Work out the finished part from the listing and answer in its coordinate system (mm). Face numbers are marked on the shaded views. A direction names the side the tool comes from. Coordinates: 2 decimals unless noted, no trailing zeros. Order: outer loops, then holes, each group sorted by start corner. A loop starts at its lowest first (then second) coordinate and runs counter-clockwise, first axis right, second up. Notation, with made-up numbers: (89, -35.5) -> (121, -35.5) arc R7 ccw to (121, -23.5) -> close; hole circle Ø5 at (42.25, 70.25). An arc over 180 degrees is marked (long way). Write item = value, one per line. Start each with the question number.
Q1. For a pull along Y with two mould halves and no side action, classify the marked faces 1, 2 and 3 as +Y half, -Y half, draft (parallel to the pull), parting line (faces both ways), or undercut.
Q2. The part is cut by section C-C, the plane x = 7.5. Count the separate pieces of the cut face and the enclosed holes in it, plus the area to 3 significant figures.
Q3. The part is cut by section A-A, the plane y = -13.5. Determine the outline of the cut face in (x, z).
Q4. Flat-ended cylindrical pins translate along their axes: pin 1 (6 mm diameter, centred on y = -32.5, z = -13, fed in from +X); pin 2 (3 mm diameter, centred on x = 7, y = -23.5, fed in from -Z). Find the tip coordinate at first contact, or state that the pin passes through.
Q5. The part is cut by section B-B, the plane y = -24. Determine the outline of the cut face in (x, z).
Q6. Which of the six approach directions +Z, -Z, +X, -X, +Y, -Y give full straight-line access (tool end or side, diameter ignored) to the marked faces 4, 5 and 6?
Q7. Straight lines are drawn through the part: L1, parallel to X at y = -25, z = -27.75; L2, parallel to Y at x = 7.5, z = -27.25; L3, parallel to Y at x = 8.5, z = -26.5. For each, find the intervals that lie inside material, in ascending order. Write a range as from..to.
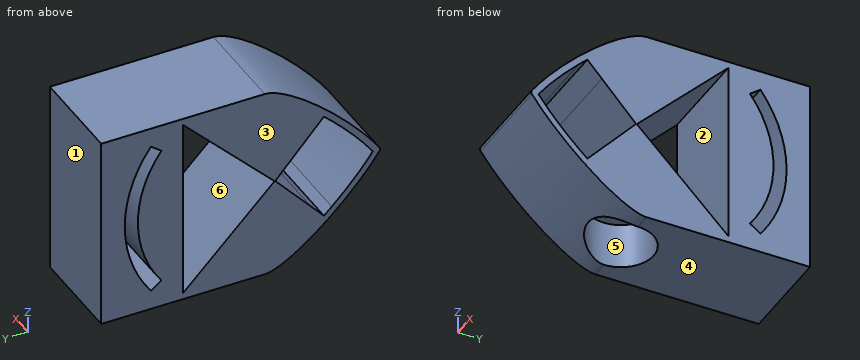
```python
from build123d import *

# Parameters (mm, degrees)
SKETCH3_W           = 30
SKETCH3_H           = 45
BOSS_EXTRUDE1_DEPTH = 15
FILLET1_SIZE        = 20
CUT_EXTRUDE3_DEPTH  = 55.331916325
CUT_EXTRUDE8_DEPTH  = 55.331916325
CUT_EXTRUDE9_DEPTH  = 55.331916325
SKETCH25_R          = 5
CUT_EXTRUDE11_DEPTH = 7
FILLET2_R           = 0.5


with BuildPart() as part:
    # Sketch3 → Boss-Extrude1 (new body)
    with BuildSketch(Plane(origin=(0, 0, 0), x_dir=(0, 0, -1), z_dir=(1, 0, 0))):
        with Locations((15, -22.5)):
            Rectangle(SKETCH3_W, SKETCH3_H)
    extrude(amount=BOSS_EXTRUDE1_DEPTH)

    # Fillet1
    # a fillet whose section is not a circle: 20 mm, written as the material it takes off along each edge
    with BuildSketch(Plane(origin=(-50, -45, -30), x_dir=(0, 1, 0), z_dir=(1, 0, 0)), Plane(origin=(-50, -45, 0), x_dir=(0, 0, -1), z_dir=(1, 0, 0))) as fillet1_piece_1:
        with BuildLine():
            Bezier((FILLET1_SIZE, 0), (0, 0), (0, FILLET1_SIZE), weights=[1, 0.23570226, 1])
            Line((0, FILLET1_SIZE), (0, 0))
            Line((0, 0), (FILLET1_SIZE, 0))
        make_face()
    extrude(amount=115, mode=Mode.SUBTRACT)

    # Sketch13 → Cut-Extrude3 (cut, through all)
    with BuildSketch(Plane(origin=(15, 0, 0), x_dir=(0, 0, -1), z_dir=(1, 0, 0))):
        Polygon((1, -12.5), (29, -12.5), (15, -26.5), align=None)
    extrude(amount=-CUT_EXTRUDE3_DEPTH, mode=Mode.SUBTRACT)

    # Sketch21 → Cut-Extrude8 (cut, through all)
    with BuildSketch(Plane(origin=(15, 0, 0), x_dir=(0, 0, -1), z_dir=(1, 0, 0))):
        with BuildLine():
            Line((20.999099472, -32.017092941), (15, -26.6))
            Line((15, -26.6), (9.197837651, -31.8392914))
            Line((9.197837651, -31.8392914), (6.751716779, -34.048112747))
            add(Edge.make_bspline(
                [(6.751716779, -34.048112747), (7.137670563, -34.475530569), (7.537017115, -34.903979725), (7.94976684, -35.333427086)],
                knots=[0.510805621, 0.510805621, 0.510805621, 0.510805621, 0.58717305, 0.58717305, 0.58717305, 0.58717305], degree=3))
            add(Edge.make_bspline(
                [(7.94976684, -35.333427086), (8.154213463, -35.546144521), (8.361948556, -35.759106865), (8.74730745, -36.148443801), (8.924817998, -36.325675997), (9.632110907, -37.023426184), (10.866534028, -38.197036851), (12.552696064, -39.658637771), (13.705600922, -40.565790559), (14.17200535, -40.917925916), (14.185722754, -40.928272256), (14.211686476, -40.947827457), (14.276533102, -40.99660607), (14.547571615, -41.199178962), (14.800672356, -41.38335147), (14.999893178, -41.525081651)],
                knots=[0.58717305, 0.58717305, 0.58717305, 0.58717305, 0.625, 0.625, 0.65625, 0.65625, 0.75, 0.875, 0.95703125, 0.95703125, 0.958984375, 0.958984375, 0.9609375, 0.96875, 1, 1, 1, 1], degree=3))
            add(Edge.make_bspline(
                [(14.999893178, -41.525081651), (15.199321685, -41.383202546), (15.452729149, -41.198806282), (15.737075559, -40.986289622), (15.815081437, -40.9275387), (15.85416041, -40.898031283), (15.864256494, -40.890397912), (16.318047278, -40.547025448), (17.4556848, -39.650959263), (19.12477944, -38.204529259), (20.355024133, -37.035590602), (21.060002804, -36.340635733), (21.237350271, -36.163716309), (21.656669951, -35.740378843), (21.89625213, -35.494384393), (22.131454088, -35.24870359)],
                knots=[0, 0, 0, 0, 0.03125, 0.0390625, 0.04296875, 0.04296875, 0.044921875, 0.044921875, 0.125, 0.25, 0.34375, 0.34375, 0.375, 0.375, 0.41847678, 0.41847678, 0.41847678, 0.41847678], degree=3))
            add(Edge.make_bspline(
                [(22.131454088, -35.24870359), (22.51540209, -34.847649728), (22.88767772, -34.447431671), (23.24828941, -34.048076256)],
                knots=[0.41847678, 0.41847678, 0.41847678, 0.41847678, 0.489449076, 0.489449076, 0.489449076, 0.489449076], degree=3))
            Line((23.24828941, -34.048076256), (20.999099472, -32.017092941))
        make_face()
    extrude(amount=-CUT_EXTRUDE8_DEPTH, mode=Mode.SUBTRACT)

    # Sketch23 → Cut-Extrude9 (cut, through all)
    with BuildSketch(Plane(origin=(15, 0, 0), x_dir=(0, 0, -1), z_dir=(1, 0, 0))):
        with BuildLine():
            Line((27, -7.6), (25.8, -9.2))
            ThreePointArc((25.8, -9.2), (15, -5.6), (4.2, -9.2))
            Line((4.2, -9.2), (3, -7.6))
            ThreePointArc((3, -7.6), (15, -3.6), (27, -7.6))
        make_face()
    extrude(amount=-CUT_EXTRUDE9_DEPTH, mode=Mode.SUBTRACT)

    # Sketch25 → Cut-Extrude11 (cut)
    with BuildSketch(Plane(origin=(0, 0, -30), x_dir=(-1, 0, 0), z_dir=(0, 0, -1))):
        with Locations(Location((-7.5, -25, 0), (0, 0, 90))):
            Circle(SKETCH25_R)
    extrude(amount=-CUT_EXTRUDE11_DEPTH, mode=Mode.SUBTRACT)

    # Fillet2
    fillet2_edges = [part.edges().sort_by_distance(p)[0] for p in [
        (7.5, -42.742918852, -15),
    ]]
    fillet(fillet2_edges, radius=FILLET2_R)


solid = part.part
```
Model answer:
q1.face_1 = +Y half
q1.face_2 = undercut
q1.face_3 = draft
q2.separate_pieces = 1
q2.enclosed_holes = 3
q2.area = 634 mm2
q3.outline = (0, -30) -> (15, -30) -> (15, -28) -> (0, -28) -> close; (0, -2) -> (15, -2) -> (15, 0) -> (0, 0) -> close
q4.pin_1 = through
q4.pin_2 = -23
q5.outline = (0, -30) -> (2.6, -30) -> (2.6, -23) -> (12.4, -23) -> (12.4, -30) -> (15, -30) -> (15, -17.5) -> (0, -17.5) -> close; (0, -12.5) -> (15, -12.5) -> (15, 0) -> (0, 0) -> close
q6.face_4 = -Z, +X, -X, +Y, -Y
q6.face_5 = -Z
q6.face_6 = +X, -X
q7.L1 = 0..2.5, 12.5..15
q7.L2 = -30.71..-30, -20..-14.25, -12.5..0
q7.L3 = -31.71..-29.9, -20.1..-15, -12.5..-8.27, -7.24..0
